Work out the finished part from the listing and answer in its coordinate system (mm). A direction names the side the tool comes from. Give positions to 0.01 mm unless a question says otherwise; leave off trailing zeros. Write each loop counter-clockwise with the first axis right and the second up, starting at its lowest first coordinate (ties: lowest second). Pieces come first, ordered by that corner, then holes. Notation, with made-up numbers: (-31.75, -9.75) -> (-8.75, -9.75) arc R20 ccw to (-8.75, 2.25) -> close; hole circle Ø2 at (35, 1). An arc over 180 degrees is marked (long way). Use a Markdown table: item, result. Add a question column.
Q1. For a pull along Y with two mould halves and no side action, classify faces 4 (the face through (16.438, -14.152, 0.986)), 5 (the face through (4, -19, 2)), 6 (the face through (-3, -18.471, 1)) as pulls with the +Y half, pulls with the -Y half, needs draft (parallel to the pull), parting line crosses it, or undercut.
Q2. Section B-B, the plane y = -13 is taken. Give the vertices of the cut face in (x, z).
Q3. Each of these flat-tipped pins is pushed along its axis until it touches: pin 1 Ø1.2 at (y, z) = (-21.5, 1.5) entering from +X; pin 2 Ø4 at (x, y) = (11.65, -18.271) entering from -Z; pin 3 Ø1.2 at (y, z) = (-14.5, 1.5) entering from -X. Where does it stop, or does it pass through?
Q4. Section A-A, the plane x = 11.65 is taken. Give the vertices of the cut face in (y, z).
Q5. Consider line 1 (Y direction, x = 0, z = 1); line 2 (X direction, y = -19.75, z = 1.85); line 3 (Y direction, x = 1, z = 0.75). Determine where each line is inside the solid, lowest interval first.
Q6. Section D-D, the plane x = 3.5 is taken. Give the vertices of the cut face in (y, z).
Q7. For faces 1 (the face through (3, -18.071, 1)), 2 (the face through (-0.044, -11.162, 0.403)), 3 (the face through (-10.878, -28.997, 0.986)), determine the directions among +Z, -Z, +X, -X, +Y, -Y from which every point of the face is accessible in a straight line to the end or side of a thin tool.
Q8. Section C-C, the plane z = 1.4 is taken. Give the vertices of the cut face in (x, y), plus the area to 3 significant figures.
Autodesk Inventor part; units mm, degrees
ref_plane "YZ Plane" through (0, 0, 0) normal (1, 0, 0) x (0, 1, 0)
ref_plane "XZ Plane" through (0, 0, 0) normal (0, 1, 0) x (-1, 0, 0)
ref_plane "XY Plane" through (0, 0, 0) normal (0, 0, 1) x (1, 0, 0)
sketch "Sketch1" plane through (0, 0, 0) normal (0, 0, 1) x (1, 0, 0)
  circle A0 centre (0, 0) radius 6.5 construction
  ellipse E0 centre (0, -17.162) end of major axis (0, -11.841) minor radius 5 construction
  line L0 (0, -44.4052) -> (0, 16.7342)
  ellipse E1 centre (0, -19.38) end of major axis (0, -14.059) minor radius 5 construction
  line L1 (0, -17.162) -> (0, -19.38) construction
  line L2 (-6, -17.162) -> (-6, -19.38)
  line L3 (6, -19.38) -> (6, -17.162)
  arc A1 (6, -17.162) -> (-6, -17.162) centre (0, -17.162) ccw
  arc A2 (-6, -19.38) -> (6, -19.38) centre (0, -19.38) ccw
  circle A3 centre (0, 0) radius 8 construction
  circle A4 centre (11.65, -18.271) radius 1.65
  line L4 (11.65, -18.271) -> (6, -18.271) construction
  circle A5 centre (-11.65, -18.271) radius 1.65
  line L5 (7.029, -18.271) -> (-7.029, -18.271) construction
  line L6 (7.029, -28.542) -> (-7.029, -28.542)
  line L7 (-7.029, -8) -> (7.029, -8)
  arc A6 (7.029, -28.542) -> (7.029, -8) centre (7.029, -18.271) ccw
  arc A7 (-7.029, -8) -> (-7.029, -28.542) centre (-7.029, -18.271) ccw
  circle A8 centre (0, -30) radius 1.65
  circle A9 centre (0, -25.4) radius 10.271
  line L8 (-14.3428, -25.4822) -> (-7.3138, -32.6112)
  line L9 (7.3138, -32.6112) -> (14.3428, -25.4822)
  line L10 (11.65, -18.271) -> (0, 0) construction
  point P0 (0, -18.271)
  point P1 (0, -8)
  point P2 (-0.7725, -28.542)
  point P3 (0.7725, -28.542)
  dimension "d7" = 5
  dimension "d8" = 5.321
  dimension "d10" = 5.321
  dimension "d11" = 5
  dimension "d0" = 13
  dimension "d9" = 17.162
  dimension "d12" = 2.218
  dimension "d13" = 12
  dimension "d14" = 1.5
  dimension "d15" = 3.3
  dimension "d16" = 4
  dimension "d17" = 4
  dimension "d18" = 3.3
  dimension "d19" = 4
  dimension "d50" = 3.3
  dimension "d51" = 30
  dimension "d52" = 4.6
  dimension "d54" = 21.6691
  dimension "d55" = 32.523
extrude "Extrusion3" add sketch "Sketch1" along normal blind 2 contours A9 A7 L6 A8 L0 | L0 A8 L6 A6 A9 | L8 A7 A9 | A9 A6 L9 | L6 A7 A9 A1 L2 A2 L0 A8 | A7 L7 L0 A1 A9 | A9 A1 L0 L7 A6 | A6 L6 A8 L0 A2 L3 A1 A9
sketch "Sketch4" plane through (0, 0, 2) normal (0, 0, 1) x (1, 0, 0)
  line L0 (6, -17.162) -> (6, -19.38)
  line L1 (6, -18.471) -> (-6, -18.471)
  line L2 (6, -18.071) -> (-6, -18.071)
  line L3 (6, -18.271) -> (-6, -18.271) construction
  line L4 (-6, -19.38) -> (-6, -17.162) construction
  line L5 (0.2, -11.1653) -> (0.2, -25.3767)
  arc A0 (6, -17.162) -> (-6, -17.162) centre (0, -17.162) ccw
  line L6 (-0.2, -11.1653) -> (-0.2, -25.3767)
  line L7 (0, -42.8052) -> (0, 7.1342)
  arc A1 (-6, -19.38) -> (6, -19.38) centre (0, -19.38) ccw
  arc A2 (-7.029, -8) -> (-14.3428, -25.4822) centre (-7.029, -18.271) ccw
  arc A3 (14.3428, -25.4822) -> (7.029, -8) centre (7.029, -18.271) ccw
  line L8 (7.029, -8) -> (-7.029, -8)
  arc A4 (6, -17.162) -> (-6, -17.162) centre (0, -17.162) ccw
  line L9 (6, -17.162) -> (6, -19.38)
  arc A5 (-6, -19.38) -> (6, -19.38) centre (0, -19.38) ccw
  line L10 (-6, -19.38) -> (-6, -17.162)
  circle A6 centre (-11.65, -18.271) radius 1.65
  circle A7 centre (11.65, -18.271) radius 1.65
  line L11 (-14.3428, -25.4822) -> (-7.3138, -32.6112)
  arc A8 (-7.3138, -32.6112) -> (7.3138, -32.6112) centre (0, -25.4) ccw
  line L12 (7.3138, -32.6112) -> (14.3428, -25.4822)
  point P0 (0, 0)
  point P1 (-6, -18.471)
  point P2 (-0.2, -18.471)
  point P3 (0.2, -18.471)
  point P4 (0.2, -18.071)
  point P5 (-6, -18.071)
  point P6 (-0.2, -18.071)
  dimension "d22" = 0.4
  dimension "d23" = 0.4
extrude "Extrusion4" add sketch "Sketch4" against normal blind 1.5 contours L0 L2 L5 A0 | L0 A1 L5 L1 | L6 L2 L10 A0 | L6 A1 L10 L1
chamfer "Chamfer1" distance 0.7 angle 45 5 edges at (10, -18.271, 0) (-13.3, -18.271, 0) (-0.8509, -31.4137, 0) (0, -28.35, 0) (1.4137, -29.1491, 0)
sketch "Sketch5" plane through (0, 0, 0) normal (0, 0, -1) x (-1, 0, 0)
  line L0 (-19.5, -6.271) -> (19.5, -6.271)
  line L1 (19.5, -6.271) -> (19.5, -30.271)
  line L2 (19.5, -30.271) -> (-19.5, -30.271)
  line L3 (-19.5, -30.271) -> (-19.5, -6.271)
  line L4 (-19.5, -6.271) -> (19.5, -30.271) construction
  line L5 (19.5, -6.271) -> (-19.5, -30.271) construction
  line L6 (7.029, -28.542) -> (-7.029, -28.542)
  line L7 (-7.029, -8) -> (7.029, -8)
  arc A0 (14.3428, -25.4822) -> (7.029, -8) centre (7.029, -18.271) ccw
  line L8 (0, -42.8052) -> (0, 7.1342)
  line L9 (6, -18.471) -> (0.2, -18.471) construction
  line L10 (-0.2, -18.071) -> (0.2, -18.471) construction
  line L11 (-0.2, -25.3767) -> (-0.2, -18.471) construction
  line L12 (-0.2, -18.471) -> (0.2, -18.071) construction
  line L13 (19.5, -30.271) -> (15.6547, -34.171)
  line L14 (15.6547, -34.171) -> (-15.6547, -34.171)
  line L15 (-15.6547, -34.171) -> (-19.5, -30.271)
  line L16 (-7.3138, -32.6112) -> (-14.3428, -25.4822)
  line L17 (14.3428, -25.4822) -> (7.3138, -32.6112)
  arc A1 (-7.3138, -32.6112) -> (7.3138, -32.6112) centre (0, -25.4) ccw
  point P0 (0, 0)
  point P1 (0, -18.271)
  point P2 (0, -18.271)
  point P3 (0, -18.271)
  dimension "d36" = 24
  dimension "d37" = 39
  dimension "d53" = 1.5
sketch "Sketch8" plane through (0, 0, 2) normal (0, 0, 1) x (1, 0, 0)
  line L0 (-0.2, -11.1653) -> (-0.2, -18.071)
  line L1 (-0.2, -18.071) -> (-6, -18.071)
  line L2 (-6, -18.071) -> (-6, -18.471)
  line L3 (-6, -18.471) -> (-0.2, -18.471)
  line L4 (-0.2, -18.471) -> (-0.2, -25.3767)
  arc A0 (-0.2, -25.3767) -> (0.2, -25.3767) centre (0, -19.38) ccw
  line L5 (0.2, -25.3767) -> (0.2, -18.471)
  line L6 (0.2, -18.471) -> (6, -18.471)
  line L7 (6, -18.471) -> (6, -18.071)
  line L8 (6, -18.071) -> (0.2, -18.071)
  line L9 (0.2, -18.071) -> (0.2, -11.1653)
  arc A1 (0.2, -11.1653) -> (-0.2, -11.1653) centre (0, -17.162) ccw
  line L10 (0.2, -18.471) -> (0.2, -25.3767)
  arc A2 (-0.2, -25.3767) -> (0.2, -25.3767) centre (0, -19.38) ccw
  line L11 (-0.2, -25.3767) -> (-0.2, -18.471)
  line L12 (-0.2, -18.471) -> (-6, -18.471)
  line L13 (-6, -18.471) -> (-6, -18.071)
  line L14 (-6, -18.071) -> (-0.2, -18.071)
  line L15 (-0.2, -18.071) -> (-0.2, -11.1653)
  arc A3 (0.2, -11.1653) -> (-0.2, -11.1653) centre (0, -17.162) ccw
  line L16 (0.2, -11.1653) -> (0.2, -18.071)
  line L17 (0.2, -18.071) -> (6, -18.071)
  line L18 (6, -18.071) -> (6, -18.471)
  line L19 (6, -18.471) -> (0.2, -18.471)
  line L20 (-0.2, -11.1653) -> (-0.2, -11.1653)
  arc A4 (0.2, -11.1653) -> (-0.2, -11.1653) centre (0, -17.162) ccw
  line L21 (0.2, -11.1653) -> (0.2, -11.1653)
  line L22 (0.2, -25.3767) -> (0.2, -25.3767)
  line L23 (-0.2, -25.3767) -> (-0.2, -25.3767)
  line L24 (-6, -18.471) -> (-6, -18.471)
  line L25 (-6, -18.071) -> (-6, -18.471)
  line L26 (-6, -18.071) -> (-6, -18.071)
  line L27 (6, -18.071) -> (6, -18.071)
  line L28 (6, -18.471) -> (6, -18.471)
  point P0 (0, 0)
  dimension "d47" = 0.4
sketch "Sketch6" plane through (-6, 6.479, 2) normal (0, 0, 1) x (1, 0, 0)
  line L0 (5.25, 6.3119) -> (5.25, 0)
  line L1 (5.25, 0) -> (0, 0)
  line L2 (0, 0) -> (0, -1.5)
  line L3 (0, -1.5) -> (5.25, -1.5)
  line L4 (5.25, -1.5) -> (5.25, -7.8119)
  arc A0 (5.25, -7.8119) -> (6.75, -7.8119) centre (6, -1.859) ccw
  line L5 (6.75, -7.8119) -> (6.75, -1.5)
  line L6 (6.75, -1.5) -> (12, -1.5)
  line L7 (12, -1.5) -> (12, 0)
  line L8 (12, 0) -> (6.75, 0)
  line L9 (6.75, 0) -> (6.75, 6.3119)
  arc A1 (6.75, 6.3119) -> (5.25, 6.3119) centre (6, 0.359) ccw
  line L10 (6.5, -0.25) -> (11.75, -0.25)
  line L11 (11.75, -0.25) -> (11.75, -1.25)
  line L12 (11.75, -1.25) -> (6.5, -1.25)
  line L13 (6.5, -1.25) -> (6.5, -7.5872)
  arc A2 (5.5, -7.5872) -> (6.5, -7.5872) centre (6, -1.859) ccw
  line L14 (5.5, -7.5872) -> (5.5, -1.25)
  line L15 (5.5, -1.25) -> (0.25, -1.25)
  line L16 (0.25, -1.25) -> (0.25, -0.25)
  line L17 (0.25, -0.25) -> (5.5, -0.25)
  line L18 (5.5, -0.25) -> (5.5, 6.0872)
  arc A3 (6.5, 6.0872) -> (5.5, 6.0872) centre (6, 0.359) ccw
  line L19 (6.5, 6.0872) -> (6.5, -0.25)
  point P0 (6, -6.479)
  dimension "d41" = 0.25
sketch "Sketch7" plane through (0, 0, 2) normal (0, 0, 1) x (1, 0, 0)
  line L0 (18.2501, 17.0189) -> (18.2501, 11.7049) construction
  line L1 (18.2501, 11.7049) -> (11.9326, 11.7049) construction
  line L2 (11.9326, 11.7049) -> (11.9326, 17.0189) construction
  line L3 (11.9326, 17.0189) -> (18.2501, 17.0189) construction
  line L4 (-15.246, -25.6115) -> (-15.246, -29.9114) construction
  line L5 (-15.246, -29.9114) -> (-18.746, -29.9114) construction
  line L6 (-18.746, -29.9114) -> (-18.746, -25.6115) construction
  line L7 (-18.746, -25.6115) -> (-15.246, -25.6115) construction
  point P0 (0, 0)
equation "\"d10\" = d8"
equation "\"d11\" = d7"
equation "\"d17\" = d16"
equation "\"d18\" = d15"
equation "\"d50\" = d15"
equation "\"d23\" = d22"
properties part number "Cover" material "Rubber"
Result set:
| question | item | result |
|---|---|---|
| 1 | face 4 | parting line crosses it |
| 1 | face 5 | needs draft |
| 1 | face 6 | undercut |
| 2 | outline | (-15.84, 0) -> (-4.32, 0) -> (-4.32, 0.5) -> (-0.2, 0.5) -> (-0.2, 2) -> (-15.84, 2) -> close; (0.2, 0.5) -> (4.32, 0.5) -> (4.32, 0) -> (15.84, 0) -> (15.84, 2) -> (0.2, 2) -> close |
| 3 | pin 1 | stops at x = 16.96 |
| 3 | pin 2 | stops at z = 0.35 |
| 3 | pin 3 | stops at x = -16.8 |
| 4 | outline | (-28.21, 0) -> (-20.62, 0) -> (-19.92, 0.7) -> (-19.92, 2) -> (-28.21, 2) -> close; (-16.62, 0.7) -> (-15.92, 0) -> (-9.1, 0) -> (-9.1, 2) -> (-16.62, 2) -> close |
| 5 | line 1 | y = -35.67 to -31.65, -28.35 to -25.38, -11.16 to -8 |
| 5 | line 2 | x = -17.19 to -12.38, -10.92 to -0.2, 0.2 to 10.92, 12.38 to 17.19 |
| 5 | line 3 | y = -35.62 to -31.31, -28.69 to -18.47, -18.07 to -8 |
| 6 | outline | (-35.06, 0) -> (-24.25, 0) -> (-24.25, 0.5) -> (-18.47, 0.5) -> (-18.47, 2) -> (-35.06, 2) -> close; (-18.07, 0.5) -> (-12.29, 0.5) -> (-12.29, 0) -> (-8, 0) -> (-8, 2) -> (-18.07, 2) -> close |
| 7 | face 1 | +Z, -Z |
| 7 | face 2 | -Z |
| 7 | face 3 | +Z, -Z, -X, -Y |
| 8 | outline | (-14.34, -25.48) -> (-7.31, -32.61) arc R10.27 ccw to (7.31, -32.61) -> (14.34, -25.48) arc R10.27 ccw to (7.03, -8) -> (-7.03, -8) arc R10.27 ccw to start; hole circle Ø3.3 at (-11.65, -18.27); hole (-6, -18.47) -> (-0.2, -18.47) -> (-0.2, -25.38) arc R6 ccw to (0.2, -25.38) -> (0.2, -18.47) -> (6, -18.47) -> (6, -18.07) -> (0.2, -18.07) -> (0.2, -11.17) arc R6 ccw to (-0.2, -11.17) -> (-0.2, -18.07) -> (-6, -18.07) -> close; hole circle Ø3.3 at (0, -30); hole circle Ø3.3 at (11.65, -18.27) |
| 8 | area | 696 mm2 |
